from build123d import *

# Parameters (mm, degrees)
SKETCH1_R           = 1.75
BOSS_EXTRUDE1_DEPTH = 4
SKETCH2_W           = 12.132955251
SKETCH2_H           = 30.105
CUT_EXTRUDE2_DEPTH  = 1


with BuildPart() as part:
    # Sketch1 → Boss-Extrude1 (new body)
    with BuildSketch(Plane.XY):
        with BuildLine():
            Line((22.242640687, -103.68381275), (30.337922061, -95.588531376))
            ThreePointArc((30.337922061, -95.588531376), (33.58215555, -93.420803863), (37.408989873, -92.659599188))
            Line((37.408989873, -92.659599188), (97.386933012, -92.659599188))
            Line((97.386933012, -92.659599188), (98.455, -92.659599188))
            ThreePointArc((98.455, -92.659599188), (99.869213562, -92.07381275), (100.455, -90.659599188))
            Line((100.455, -90.659599188), (100.455, -24.874599188))
            ThreePointArc((100.455, -24.874599188), (99.869213562, -23.460385626), (98.455, -22.874599188))
            Line((98.455, -22.874599188), (97.38733653, -22.874599188))
            Line((97.38733653, -22.874599188), (37.403989873, -22.874599188))
            ThreePointArc((37.403989873, -22.874599188), (33.57715555, -22.113394513), (30.332922061, -19.945667))
            Line((30.332922061, -19.945667), (22.242640687, -11.855385626))
            ThreePointArc((22.242640687, -11.855385626), (21.593793989, -11.421840123), (20.828427125, -11.269599188))
            Line((20.828427125, -11.269599188), (-16.3, -11.269599188))
            ThreePointArc((-16.3, -11.269599188), (-17.714213562, -11.855385626), (-18.3, -13.269599188))
            Line((-18.3, -13.269599188), (-18.3, -29.968425088))
            add(Edge.make_bspline(
                [(-18.3, -29.968425088), (-18.3, -30.568817376), (-18.296844416, -31.1692069), (-18.296844416, -31.769599188), (-18.296844416, -32.369991476), (-18.3, -32.970381), (-18.3, -33.570773288)],
                knots=[0, 0, 0, 0, 0.001801177, 0.001801177, 0.001801177, 0.003602354, 0.003602354, 0.003602354, 0.003602354], degree=3))
            Line((-18.3, -33.570773288), (-18.3, -55.968425088))
            add(Edge.make_bspline(
                [(-18.3, -55.968425088), (-18.3, -56.568817376), (-18.296844416, -57.1692069), (-18.296844416, -57.769599188), (-18.296844416, -58.369991476), (-18.3, -58.970381), (-18.3, -59.570773288)],
                knots=[0, 0, 0, 0, 0.001801177, 0.001801177, 0.001801177, 0.003602354, 0.003602354, 0.003602354, 0.003602354], degree=3))
            Line((-18.3, -59.570773288), (-18.3, -81.968425088))
            add(Edge.make_bspline(
                [(-18.3, -81.968425088), (-18.3, -82.568817376), (-18.296844416, -83.1692069), (-18.296844416, -83.769599188), (-18.296844416, -84.369991476), (-18.3, -84.970381), (-18.3, -85.570773288)],
                knots=[0, 0, 0, 0, 0.001801177, 0.001801177, 0.001801177, 0.003602354, 0.003602354, 0.003602354, 0.003602354], degree=3))
            Line((-18.3, -85.570773288), (-18.3, -102.269599188))
            ThreePointArc((-18.3, -102.269599188), (-17.714213562, -103.68381275), (-16.3, -104.269599188))
            Line((-16.3, -104.269599188), (20.828427125, -104.269599188))
            ThreePointArc((20.828427125, -104.269599188), (21.593793989, -104.117358253), (22.242640687, -103.68381275))
        make_face()
        with Locations((-15.716636906, -101.686236094)):
            Circle(SKETCH1_R, mode=Mode.SUBTRACT)
        with Locations((-15.716636906, -13.852962283)):
            Circle(SKETCH1_R, mode=Mode.SUBTRACT)
        with Locations((32.622607905, -24.417876383)):
            Circle(SKETCH1_R, mode=Mode.SUBTRACT)
        with Locations((32.627607905, -91.116321993)):
            Circle(SKETCH1_R, mode=Mode.SUBTRACT)
        with Locations((97.869213562, -90.07381275)):
            Circle(SKETCH1_R, mode=Mode.SUBTRACT)
        with Locations((97.869213562, -25.460385626)):
            Circle(SKETCH1_R, mode=Mode.SUBTRACT)
    extrude(amount=BOSS_EXTRUDE1_DEPTH)

    # Sketch2 → Cut-Extrude2 (cut)
    with BuildSketch(Plane(origin=(0, 0, 0), x_dir=(-1, 0, 0), z_dir=(0, 0, -1))):
        with Locations((-74.209835266, -56.927099188)):
            Rectangle(SKETCH2_W, SKETCH2_H)
    extrude(amount=-CUT_EXTRUDE2_DEPTH, mode=Mode.SUBTRACT)


solid = part.part
Model file for the job. Use its own axes, mm. A direction names the side the tool comes from. Give positions to 0.01 mm unless a question says otherwise; leave off trailing zeros. Order: outer loops, then holes, each group sorted by start corner. A loop starts at its lowest first (then second) coordinate and runs counter-clockwise, first axis right, second up. Notation, with made-up numbers: (31.5, -27.75) - (45.5, -27.75) arc R16 cw to (45.5, -20.75) - close; hole circle Ø8 at (71, 33). An arc over 180 degrees is marked (long way). Write item = value, one per line. Start each with the question number.
1. Drop flat-ended pins along their axis: P1, Ø1, axis at y = -23, z = 0.5, coming from the +X side; P2, Ø3, axis at x = -15.72, y = -101.69, coming from the -Z side; P3, Ø0.5, axis at x = 76, z = 0.5, coming from the -Y side; P4, Ø1.5, axis at y = -91.5, z = 1, coming from the +X side. Give the stop position or say it passes through.
2. Cut at B-B, the plane x = 81.5. List the corners of the cut face in (y, z).
3. Which spindle directions (+Z, -Z, +X, -X, +Y, -Y) get a long thin tool onto all of the face, cutting with end or side? Do faces 1 (the flat face through (68, -22.875, 2)), 2 (the flat face through (68, -92.66, 2)), 3 (the cylindrical face through (96.12, -25.38, 1.97)), 4 (the flat face through (74, -57, 1)). Say none if no direction does.
4. Cut at C-C, the plane z = 3. State how many separate pieces and enclosed holes the cut face has, and give its area (3 significant figures).
5. Probe line 1 along X through (y, z) = (-90, 1.85) (3 decimals); line 2 along Y through (x, z) = (78.5, 0.45); line 3 along X through (y, z) = (-91.5, 0.8). List the from-to ranges inside material, lowest first.
6. Two-plate mould, pull along X, no slides. Class faces 5 (the flat face through (-18.3, -94, 2)), 6 (the cylindrical face through (-17.465, -13.776, 1.972)), 7 (the flat face through (26.344, -15.957, 1.972)), 8 (the flat face through (3, -11.27, 2)): pulls with the +X half, pulls with the -X half, needs draft (parallel to the pull), parting line crosses it, or undercut.
7. Cut at A-A, the plane y = -52. List the corners of the cut face in (x, z) (3 decimals).
Taken from the geometry:
q1.P1 = 99.91
q1.P2 = through
q1.P3 = -92.66
q1.P4 = 100.45
q2.outline = (-92.66, 0) - (-22.87, 0) - (-22.87, 4) - (-92.66, 4) - close
q3.face_1 = +Z, -Z, +X, +Y
q3.face_2 = +Z, -Z, +X, -Y
q3.face_3 = +Z, -Z
q3.face_4 = -Z
q4.separate_pieces = 1
q4.enclosed_holes = 6
q4.area = 9,290 mm²
q5.line_1 = -18.3 to 31.28, 33.975 to 96.121, 99.618 to 100.455
q5.line_2 = -92.66 to -71.98, -41.87 to -22.87
q5.line_3 = -18.3 to 30.92, 34.34 to 96.86, 98.88 to 100.27
q6.face_5 = pulls with the -X half
q6.face_6 = undercut
q6.face_7 = pulls with the +X half
q6.face_8 = needs draft
q7.outline = (-18.3, 0) - (68.143, 0) - (68.143, 1) - (80.276, 1) - (80.276, 0) - (100.455, 0) - (100.455, 4) - (-18.3, 4) - close
